The model under review builds one solid part; all positions refer to its coordinate system, in mm. Face numbers are marked on the shaded views. Round coordinates to 2 decimals unless told otherwise and drop trailing zeros. Write each loop counter-clockwise with the first axis right and the second up, starting at its lowest first coordinate (ties: lowest second). Pieces come first, ordered by that corner, then holes. Notation, with made-up numbers: M -4.5,50.25 L 14.5,50.25 A34 cw 14.5,85.25 Z; hole C 16.5,17 d6. An arc over 180 degrees is marked long. One line per item, written item: value. Start each with the question number.
1) For P1, Ø3.5, axis at x = 10, y = 30.75, coming from the -Z side; P2, Ø3, axis at y = -27, z = 4, coming from the +X side, all flat-tipped, find the tip position at first contact; note any pin that passes through.
2) Take a section at A-A, the plane y = 30.75. Write out the cut boundary in (x, z), and give its area (3 significant figures).
3) Take a section at C-C, the plane z = 4.2. Write out the cut boundary in (x, y).
4) Take a section at B-B, the plane x = 3.5. Write out the cut boundary in (y, z).
5) Take a section at D-D, the plane x = -16. Write out the cut boundary in (y, z).
6) Wall thickness on probe 1 along Y at (x, z) = (0, 5.85); probe 2 along Y at (x, z) = (-12, 3.2); probe 3 along X at (y, z) = (-24, 2.8): over which ranges is each line inside the solid? List them lowest first.
7) Mouldability with a two-part tool opening along Y and no side actions: class the marked faces 1, 2, 3 and 4 as +Y half, -Y half, draft (parallel to the pull), parting line (faces both ways), or undercut.
Autodesk Inventor part; units mm, degrees
ref_plane "YZ Plane" through (0, 0, 0) normal (1, 0, 0) x (0, 1, 0)
ref_plane "XZ Plane" through (0, 0, 0) normal (0, 1, 0) x (-1, 0, 0)
ref_plane "XY Plane" through (0, 0, 0) normal (0, 0, 1) x (1, 0, 0)
sketch "Sketch1" plane through (0, 0, 0) normal (0, 0, 1) x (1, 0, 0)
  arc A0 (-19.25, -19.25) -> (19.25, -19.25) centre (0, -19.25) ccw
  circle A1 centre (0, -19.25) radius 10.5
  arc A2 (11.9852, -26.1697) -> (14.1148, -27.3992) centre (13.05, -26.7844) ccw
  arc A3 (-11.9852, -26.1697) -> (-14.1148, -27.3992) centre (-13.05, -26.7844) ccw
  arc A4 (0, -5.4107) -> (0, -2.9517) centre (0, -4.1812) ccw
  line L0 (0, -19.25) -> (14.5554, -15.3499) construction
  line L1 (0, -19.25) -> (13.05, -26.7844) construction
  line L2 (0, -19.25) -> (-10.6553, -8.5947) construction
  line L3 (0, -19.25) -> (0, -4.1812) construction
  line L4 (0, -19.25) -> (-3.9001, -33.8054) construction
  line L5 (0, -19.25) -> (-13.05, -26.7844) construction
  arc A5 (-4.2183, -34.993) -> (-3.5819, -32.6178) centre (-3.9001, -33.8054) ccw
  arc A6 (15.743, -15.0317) -> (13.3678, -15.6681) centre (14.5554, -15.3499) ccw
  arc A7 (-11.5247, -7.7253) -> (-9.7859, -9.4641) centre (-10.6553, -8.5947) ccw
  arc A8 (0, -2.9517) -> (-11.5247, -7.7253) centre (0, -19.25) ccw
  arc A9 (0, -5.4107) -> (-9.7859, -9.4641) centre (0, -19.25) ccw
  arc A10 (11.9852, -26.1697) -> (13.3678, -15.6681) centre (0, -19.25) ccw
  arc A11 (14.1148, -27.3992) -> (15.743, -15.0317) centre (0, -19.25) ccw
  arc A12 (-11.9852, -26.1697) -> (-3.5819, -32.6178) centre (0, -19.25) ccw
  arc A13 (-14.1148, -27.3992) -> (-4.2183, -34.993) centre (0, -19.25) ccw
  line L6 (19.25, -19.25) -> (19.25, 42.75)
  line L7 (-19.25, -19.25) -> (-19.25, 42.75)
  line L8 (19.25, 42.75) -> (-19.25, 42.75)
  circle A14 centre (-10, 30.75) radius 2.25
  circle A15 centre (10, 30.75) radius 2.25
  line L9 (10, 30.75) -> (-10, 30.75)
  point P0 (0, 0)
  point P1 (19.25, 30.75)
  dimension "d0" = 21
  dimension "d1" = 45
  dimension "d2" = 45
  dimension "d3" = 45
  dimension "d4" = 2.459
  dimension "d5" = 2.459
  dimension "d6" = 2.459
  dimension "d7" = 2.459
  dimension "d8" = 2.459
  dimension "d9" = 2.459
  dimension "d11" = 62
  dimension "d14" = 19.25
  dimension "d21" = 4.5
  dimension "d22" = 12
  dimension "d23" = 4.5
  dimension "d24" = 20
  dimension "d25" = 9.25
  dimension "d26" = 38.5
extrude "Extrusion1" add sketch "Sketch1" along normal blind 6
equation "\"d8\" = d6"
equation "\"d9\" = d7"
equation "\"d23\" = d21"
equation "\"d25\" = -0.5 * d24 + 0.5 * d26"
properties part number "Joint1C_1" material "PET Plastic"
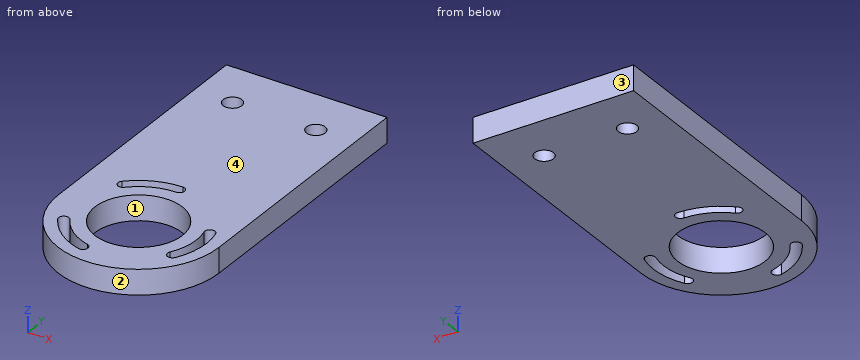
Checked values:
1. P1: passes through
1. P2: stops at x = 18.21
2. outline: M -19.25,0 L -12.25,0 L -12.25,6 L -19.25,6 Z; M -7.75,0 L 7.75,0 L 7.75,6 L -7.75,6 Z; M 12.25,0 L 19.25,0 L 19.25,6 L 12.25,6 Z
2. area: 177 mm2
3. outline: M -19.25,-19.25 A19.25 ccw 19.25,-19.25 L 19.25,42.75 L -19.25,42.75 Z; hole M -14.11,-27.4 A16.3 ccw -4.22,-34.99 A1.23 ccw -3.58,-32.62 A13.84 cw -11.99,-26.17 A1.23 ccw Z; hole C -10,30.75 d4.5; hole M -11.52,-7.73 A1.23 ccw -9.79,-9.46 A13.84 cw 0,-5.41 A1.23 ccw 0,-2.95 A16.3 ccw Z; hole C 0,-19.25 d21; hole C 10,30.75 d4.5; hole M 11.99,-26.17 A1.23 ccw 14.11,-27.4 A16.3 ccw 15.74,-15.03 A1.23 ccw 13.37,-15.67 A13.84 cw Z
4. outline: M -38.18,0 L -29.15,0 L -29.15,6 L -38.18,6 Z; M -9.35,0 L 42.75,0 L 42.75,6 L -9.35,6 Z
5. outline: M -29.95,0 L 42.75,0 L 42.75,6 L -29.95,6 Z
6. probe 1: y = -38.5 to -29.75, -8.75 to -5.41, -2.95 to 42.75
6. probe 2: y = -34.3 to -30.28, -26.14 to 29.72, 31.78 to 42.75
6. probe 3: x = -18.65 to -9.36, 9.36 to 13, 15.59 to 18.65
7. face 1: undercut
7. face 2: -Y half
7. face 3: +Y half
7. face 4: draft
